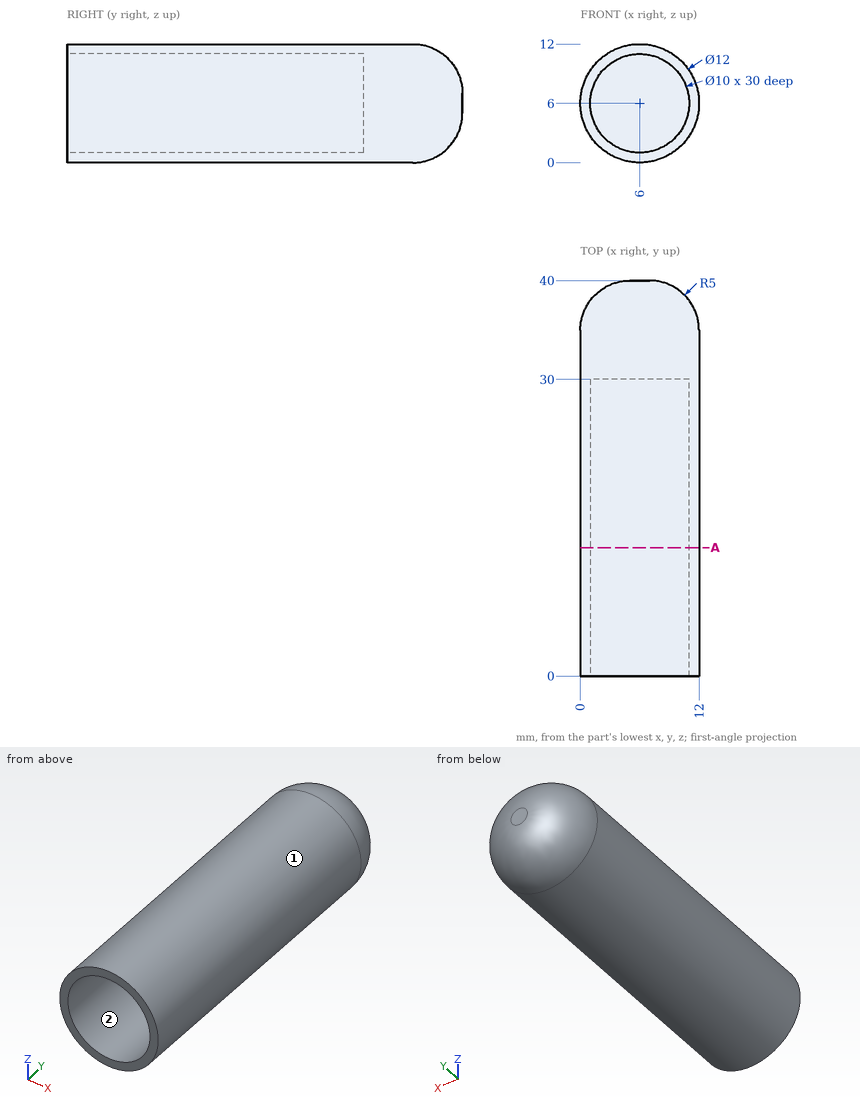
Here's the drawing with two shaded views (mm, measured from the low corner). I have some questions. Coordinates: 2 decimals unless noted, no trailing zeros. Order: outer loops, then holes, each group sorted by start corner. A loop starts at its lowest first (then second) coordinate and runs counter-clockwise, first axis right, second up.
Q1. Please list where these lines run through material, in increasing order: L1, parallel to X at y = 10.75, z = 6; L2, parallel to Z at x = 5.75, y = 6; L3, parallel to Z at x = 4.5, y = 9.5.
Q2. Suppose I cut it at A-A on y = 13. Please give me the cut outline in (x, z), and give its area (3 significant figures).
Q3. Will these pins go through, and if not, where does the flat tip stop? pin 1 (6 mm diameter, centred on x = 10.5, z = 8, fed in from +Y); pin 2 (1.5 mm diameter, centred on y = 29, z = 2, fed in from +X); pin 3 (3 mm diameter, centred on x = 6.5, z = 7.5, fed in from -Y).
Q4. Thinking about a two-plate mould opening in X: for the marked faces 1 and 2, which applies, released by +X, released by -X, zero draft, split by the parting line, or undercut?
Answer:
1. L1: x = 0 to 1, 11 to 12
1. L2: z = 0.01 to 1.01, 10.99 to 11.99
1. L3: z = 0.19 to 1.23, 10.77 to 11.81
2. outline: circle Ø12 at (6, 6); hole circle Ø10 at (6, 6)
2. area: 34.6 mm2
3. pin 1: stops at y = 39.91
3. pin 2: stops at x = 11.04
3. pin 3: stops at y = 30
4. face 1: split by the parting line
4. face 2: undercut
